from build123d import *

# Parameters (mm, degrees)
CROQUIS1_W              = 20
CROQUIS1_H              = 30
SALIENTE_EXTRUIR1_DEPTH = 1.15
CROQUIS2_W              = 8
CROQUIS2_H              = 8
SALIENTE_EXTRUIR2_DEPTH = 3
REDONDEO1_R             = 1


with BuildPart() as part:
    # Croquis1 → Saliente-Extruir1 (new body)
    with BuildSketch(Plane(origin=(0, 0, 0), x_dir=(1, 0, 0), z_dir=(0, 1, 0))):
        Rectangle(CROQUIS1_W, CROQUIS1_H)
    extrude(amount=SALIENTE_EXTRUIR1_DEPTH)

    # Croquis2 → Saliente-Extruir2 (add)
    with BuildSketch(Plane(origin=(0, 1.15, 0), x_dir=(1, 0, 0), z_dir=(0, 1, 0))):
        with Locations((0, 12)):
            Rectangle(CROQUIS2_W, CROQUIS2_H)
    extrude(amount=SALIENTE_EXTRUIR2_DEPTH)

    # Redondeo1
    redondeo1_edges = [part.edges().sort_by_distance(p)[0] for p in [
        (-4, 1.15, -15.5),
        (4, 1.15, -15.5),
        (-4, 4.15, -12),
        (4, 4.15, -12),
    ]]
    fillet(redondeo1_edges, radius=REDONDEO1_R)


solid = part.part
Design review of the part built by this model. Coordinates are the model's own, in mm. A direction names the side the tool comes from. Round coordinates to 2 decimals unless told otherwise and drop trailing zeros. Loops run counter-clockwise (first coordinate to the right, second up) from the corner with the lowest first, then second, coordinate; pieces in that order, holes last. Notation, with made-up numbers: M 67.5,48 L 113.5,48 A26 cw 113.5,71 Z; hole C 68.25,84.25 d11. An arc over 180 degrees is marked long. Answer as a JSON object with one key per item and string values.
Item 1: We need section C-C on y = 2.5. Give the boundary of the cut face in (x, z).
Answer sheet:
{"outline": "M -4,-16 L 4,-16 L 4,-8 L -4,-8 Z"}
Item 2: We need section D-D on x = -5. Give the boundary of the cut face in (y, z), and give its area (3 significant figures).
Answer sheet:
{"outline": "M 0,-15 L 1.15,-15 L 1.15,15 L 0,15 Z", "area": "34.5 mm^2"}
Item 3: Wall thickness on L1, parallel to Z at x = 5.25, y = 0.2; L2, parallel to Y at x = -2.75, z = -5; L3, parallel to X at y = 1.65, z = -8.5: over which ranges is each line inside the solid? List them lowest first. Write a range as from..to.
Answer sheet:
{"L1": "z = -15..15", "L2": "y = 0..1.15", "L3": "x = -4..4"}
Item 4: Machinability: for faces 1 (the flat face through (0, 1.15, -15.5)), 2 (the flat face through (-4, 2, -12)), 3 (the flat face through (0, 3, -8)), 4 (the cylindrical face through (-3.715, 1.451, -15.507)), which of the approach directions +Z, -Z, +X, -X, +Y, -Y give a long, thin tool a straight path to every point of the face, cutting with its end or side? Answer none if there is none.
Answer sheet:
{"face 1": "-Z, +X, -X, -Y", "face 2": "+Z, -Z, -X, +Y", "face 3": "+Z, +X, -X, +Y", "face 4": "-Z, -X, -Y"}
Item 5: We need section B-B on z = -10. Give the boundary of the cut face in (x, y).
Answer sheet:
{"outline": "M -10,0 L 10,0 L 10,1.15 L 4,1.15 L 4,3.15 A1 ccw 3,4.15 L -3,4.15 A1 ccw -4,3.15 L -4,1.15 L -10,1.15 Z"}
Item 6: We need section A-A on x = -2.25. Give the boundary of the cut face in (y, z), and give its area (3 significant figures).
Answer sheet:
{"outline": "M 0,-15 L 1.15,-15 L 1.15,-16 L 4.15,-16 L 4.15,-8 L 1.15,-8 L 1.15,15 L 0,15 Z", "area": "58.5 mm^2"}
Item 7: Clearance check with flat-ended pins moving along their axes: P1, Ø0.8, axis at x = -1, z = -15.5, coming from the -Y side; P2, Ø0.9, axis at x = -0.5, y = 2, coming from the +Z side; P3, Ø0.6, axis at y = 2.5, z = -10.5, coming from the +X side. State where each tip first meets the part, or that it passes through.
Answer sheet:
{"P1": "stops at y = 1.15", "P2": "stops at z = -8", "P3": "stops at x = 4"}
